Geometry check sheet. Reference: the model listing, model coordinates, mm. Face numbers are marked on the shaded views. A direction names the side the tool comes from. Round coordinates to 2 decimals unless told otherwise and drop trailing zeros. Write each loop counter-clockwise with the first axis right and the second up, starting at its lowest first coordinate (ties: lowest second). Pieces come first, ordered by that corner, then holes. Notation, with made-up numbers: (37, -21.5) -> (70, -21.5) arc R9 ccw to (70, -12.5) -> close; hole circle Ø3 at (24, -27.75). An arc over 180 degrees is marked (long way). Use a Markdown table: item, result.
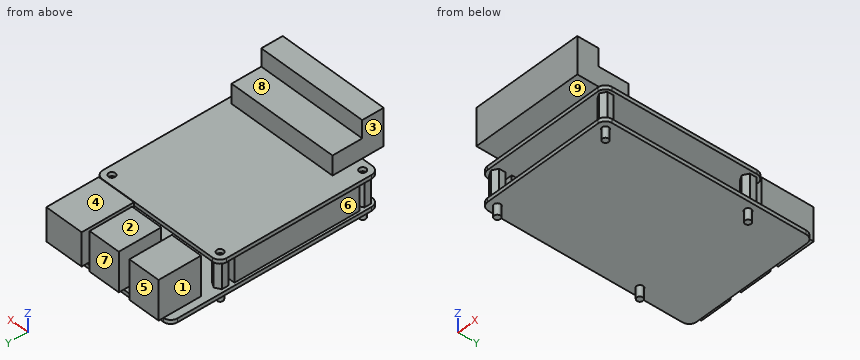
```python
from build123d import *

# Parameters (mm, degrees)
SKETCH_R     = 1.375
PAD_DEPTH    = 1.6
SKETCH001_W  = 16
SKETCH001_H  = 21.3
PAD001_DEPTH = 13.5
SKETCH002_W  = 13.2
SKETCH002_H  = 17.25
PAD002_DEPTH = 16
PAD008_DEPTH = 11
SKETCH011_R  = 1.25
PAD009_DEPTH = 6
SKETCH012_W  = 5
SKETCH012_H  = 50.8
PAD010_DEPTH = 11
SKETCH013_R  = 1.375
PAD011_DEPTH = 1.6
PAD012_DEPTH = 45.72


with BuildPart() as part:
    # Sketch → Pad (new body)
    with BuildSketch(Plane.XY):
        with BuildLine():
            ThreePointArc((-25, 42.5), (-27.12132, 41.62132), (-28, 39.5))
            Line((-28, -39.5), (-28, 39.5))
            ThreePointArc((-28, -39.5), (-27.12132, -41.62132), (-25, -42.5))
            Line((25, -42.5), (-25, -42.5))
            ThreePointArc((25, -42.5), (27.12132, -41.62132), (28, -39.5))
            Line((28, 39.5), (28, -39.5))
            ThreePointArc((28, 39.5), (27.12132, 41.62132), (25, 42.5))
            Line((-25, 42.5), (25, 42.5))
        make_face()
        with Locations((-24.5, 19)):
            Circle(SKETCH_R, mode=Mode.SUBTRACT)
        with Locations((24.5, 19)):
            Circle(SKETCH_R, mode=Mode.SUBTRACT)
        with Locations((-24.5, -39)):
            Circle(SKETCH_R, mode=Mode.SUBTRACT)
        with Locations((24.5, -39)):
            Circle(SKETCH_R, mode=Mode.SUBTRACT)
    extrude(amount=PAD_DEPTH)

    # Sketch001 → Pad001 (join)
    with BuildSketch(Plane.XY.offset(1.6)):
        with Locations((17.6, 34.05)):
            Rectangle(SKETCH001_W, SKETCH001_H)
    extrude(amount=PAD001_DEPTH)

    # Sketch002 → Pad002 (join)
    with BuildSketch(Plane.XY.offset(1.6)):
        with Locations((-18.4, 35.875)):
            Rectangle(SKETCH002_W, SKETCH002_H)
        with Locations((-0.4, 35.875)):
            Rectangle(SKETCH002_W, SKETCH002_H)
    extrude(amount=PAD002_DEPTH)

    # Sketch010 → Pad008 (join)
    with BuildSketch(Plane.XY.offset(1.6)):
        Polygon((-22.235344, -40.3075), (-22.235344, -37.6925), (-24.5, -36.385), (-26.764656, -37.6925), (-26.764656, -40.3075), (-24.5, -41.615), align=None)
        Polygon((-22.235344, 17.6925), (-22.235344, 20.3075), (-24.5, 21.615), (-26.764656, 20.3075), (-26.764656, 17.6925), (-24.5, 16.385), align=None)
        Polygon((24.5, -41.615), (26.764656, -40.3075), (26.764656, -37.6925), (24.5, -36.385), (22.235344, -37.6925), (22.235344, -40.3075), align=None)
        Polygon((24.5, 16.385), (26.764656, 17.6925), (26.764656, 20.3075), (24.5, 21.615), (22.235344, 20.3075), (22.235344, 17.6925), align=None)
    extrude(amount=PAD008_DEPTH)

    # Sketch011 → Pad009 (join)
    with BuildSketch(Plane.XY.offset(1.6)):
        with Locations((-24.5, 19)):
            Circle(SKETCH011_R)
        with Locations((-24.5, -39)):
            Circle(SKETCH011_R)
        with Locations((24.5, 19)):
            Circle(SKETCH011_R)
        with Locations((24.5, -39)):
            Circle(SKETCH011_R)
    extrude(amount=-PAD009_DEPTH)

    # Sketch012 → Pad010 (join)
    with BuildSketch(Plane.XY.offset(1.6)):
        with Locations((-24.5, -10)):
            Rectangle(SKETCH012_W, SKETCH012_H)
    extrude(amount=PAD010_DEPTH)

    # Sketch013 → Pad011 (join)
    with BuildSketch(Plane.XY.offset(12.6)):
        with BuildLine():
            ThreePointArc((-25, 22.5), (-27.12132, 21.62132), (-28, 19.5))
            Line((-28, -39.5), (-28, 19.5))
            ThreePointArc((-28, -39.5), (-27.12132, -41.62132), (-25, -42.5))
            Line((25, -42.5), (-25, -42.5))
            ThreePointArc((25, -42.5), (27.12132, -41.62132), (28, -39.5))
            Line((28, 19.5), (28, -39.5))
            ThreePointArc((28, 19.5), (27.12132, 21.62132), (25, 22.5))
            Line((-25, 22.5), (25, 22.5))
        make_face()
        with Locations((-24.5, 19)):
            Circle(SKETCH013_R, mode=Mode.SUBTRACT)
        with Locations((24.5, 19)):
            Circle(SKETCH013_R, mode=Mode.SUBTRACT)
        with Locations((-24.5, -39)):
            Circle(SKETCH013_R, mode=Mode.SUBTRACT)
        with Locations((24.5, -39)):
            Circle(SKETCH013_R, mode=Mode.SUBTRACT)
    extrude(amount=PAD011_DEPTH)

    # Sketch014 → Pad012 (join)
    with BuildSketch(Plane(origin=(-20.34, -30.45, 14.2), x_dir=(0, 1, 0), z_dir=(1, 0, 0))):
        Polygon((0, 0), (0, 7.9), (-12.1, 7.9), (-12.1, 15.1), (-20.82, 15.1), (-20.82, 0), align=None)
    extrude(amount=PAD012_DEPTH)


solid = part.part
```
(1) Access from +Z, -Z, +X, -X, +Y, -Y to the whole of each face (thin tool, end or side, straight path). Record for the marked faces 1, 2, 3, 4 and 5.
A:
| item | result |
|---|---|
| face 1 | +Z, -X, +Y |
| face 2 | +Z, +X, -X, +Y |
| face 3 | +Z, -X, -Y |
| face 4 | +Z, +X, +Y |
| face 5 | +Z, -Z, -X, +Y |
(2) Release check for a two-part mould opening along Z. For the marked faces 6, 7, 8 and 9 record: +Z half, -Z half, draft (parallel to the pull), parting line (faces both ways), or undercut.
A:
| item | result |
|---|---|
| face 6 | undercut |
| face 7 | draft |
| face 8 | +Z half |
| face 9 | -Z half |
(3) Thickness scan on line 1 (Y direction, x = 24.5, z = 13.35) (3 decimals); line 2 (Z direction, x = -12.5, y = -7); line 3 (X direction, y = 19, z = 5). Record the ranges inside material, lowest first.
A:
| item | result |
|---|---|
| line 1 | y = -42.5 to -40.375, -37.625 to 17.625, 20.375 to 22.5, 23.4 to 44.7 |
| line 2 | z = 0 to 1.6, 12.6 to 14.2 |
| line 3 | x = -26.76 to -22.24, 22.24 to 26.76 |
(4) Gauge pin test, flat ends, axial feed: pin 1 Ø4 at (x, y) = (11, -36.5) entering from -Z; pin 2 Ø6 at (x, z) = (20, 23.5) entering from +Y; pin 3 Ø1 at (x, z) = (-8.5, 0.5) entering from +Y. Record the tip position at first contact, or that the pin passes through.
A:
| item | result |
|---|---|
| pin 1 | stops at z = 0 |
| pin 2 | stops at y = -30.45 |
| pin 3 | stops at y = 42.5 |
(5) Section check A-A on x = -1.5. Record the cut outline in (y, z).
A:
| item | result |
|---|---|
| outline | (-51.27, 14.2) -> (-42.5, 14.2) -> (-42.5, 12.6) -> (22.5, 12.6) -> (22.5, 14.2) -> (-30.45, 14.2) -> (-30.45, 22.1) -> (-42.55, 22.1) -> (-42.55, 29.3) -> (-51.27, 29.3) -> close; (-42.5, 0) -> (42.5, 0) -> (42.5, 1.6) -> (44.5, 1.6) -> (44.5, 17.6) -> (27.25, 17.6) -> (27.25, 1.6) -> (-42.5, 1.6) -> close |
(6) Section check B-B on y = -13.5. Record the cut outline in (x, z), plus the area to 3 significant figures.
A:
| item | result |
|---|---|
| outline | (-28, 0) -> (28, 0) -> (28, 1.6) -> (-22, 1.6) -> (-22, 12.6) -> (28, 12.6) -> (28, 14.2) -> (-28, 14.2) -> (-28, 12.6) -> (-27, 12.6) -> (-27, 1.6) -> (-28, 1.6) -> close |
| area | 234 mm2 |
(7) Section check D-D on z = 23.5. Record the cut outline in (x, y), plus the area to 3 significant figures.
A:
| item | result |
|---|---|
| outline | (-20.34, -51.27) -> (25.38, -51.27) -> (25.38, -42.55) -> (-20.34, -42.55) -> close |
| area | 399 mm2 |
(8) Section check C-C on z = 8.5. State how many separate pieces and enclosed holes the cut face has, plus the area to 3 significant figures.
A:
| item | result |
|---|---|
| separate pieces | 8 |
| enclosed holes | 0 |
| area | 1,120 mm2 |
